The model under review builds one solid part; all positions refer to its coordinate system, in mm. Round coordinates to 2 decimals unless told otherwise and drop trailing zeros. Order: outer loops, then holes, each group sorted by start corner. A loop starts at its lowest first (then second) coordinate and runs counter-clockwise, first axis right, second up. Notation, with made-up numbers: (87, 46.5) - (119, 46.5) arc R13 cw to (119, 65.5) - close; hole circle Ø8 at (-11, -6.75). An arc over 180 degrees is marked (long way). One line per question, with ' | ' between items. Start each with the question number.
Item 1: Add section B-B on z = 19.5. State the section outline as (x, y) points.
Item 2: For L1, parallel to Z at x = 4, y = 187.5 (3 decimals); L2, parallel to X at y = 184.5, z = 3; L3, parallel to X at y = 319, z = 8, list the stretches that pass through material, from the lowest coordinate up. Write a range as [from, to].
Item 3: Insertion check: pin 1 Ø5 at (y, z) = (121.5, 12.5) entering from -X. The pin has a flat end and moves straight along its axis. Give the tip position at first contact, or say it passes through.
Item 4: Add section C-C on y = 136. State the section outline as (x, z) points (3 decimals).
Item 5: Add section A-A on y = 100. State the section outline as (x, z) points (3 decimals).
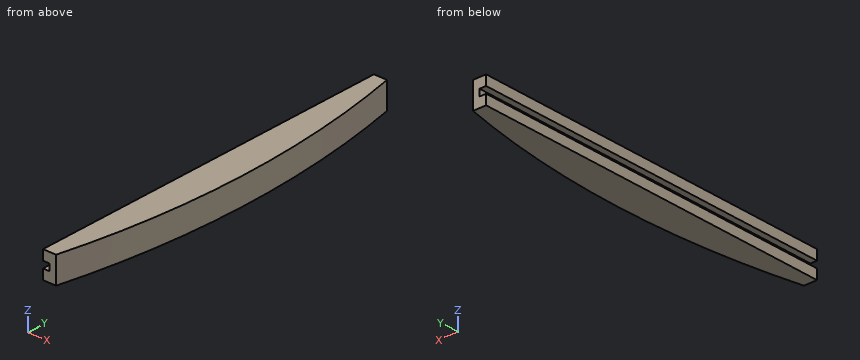
Autodesk Inventor part; units mm, degrees
ref_plane "YZ Plane" through (0, 0, 0) normal (1, 0, 0) x (0, 1, 0)
ref_plane "XZ Plane" through (0, 0, 0) normal (0, 1, 0) x (-1, 0, 0)
ref_plane "XY Plane" through (0, 0, 0) normal (0, 0, 1) x (1, 0, 0)
sketch "Sketch1" plane through (0, 0, 0) normal (0, 0, 1) x (1, 0, 0)
  line L0 (0, 0) -> (12.7, 0)
  line L1 (0, 0) -> (0, 355.8819)
  line L2 (0, 355.8819) -> (12.7, 355.8819)
  arc A0 (12.7, 0) -> (12.7, 355.8819) centre (-782.8431, 177.941) ccw
  dimension "d0" = 12.7
  dimension "d1" = 355.8819
  dimension "d2" = 12.7
extrude "Extrusion1" add sketch "Sketch1" along normal blind 25.4
sketch "Sketch2" plane through (0, 0, 0) normal (-1, 0, 0) x (0, 0, 1)
  line L0 (0, 0) -> (12.7, 0)
  line L1 (0, 0) -> (25.4, 0)
  line L2 (12.7, 355.8819) -> (9.525, 355.8819)
  line L3 (9.525, 355.8819) -> (9.525, 0)
  line L4 (9.525, 0) -> (15.875, 0)
  line L5 (15.875, 0) -> (15.875, 355.8819)
  line L6 (9.525, 355.8819) -> (15.875, 355.8819)
  line L7 (9.525, 0) -> (15.875, 0)
  dimension "d5" = 12.7
  dimension "d6" = 3.175
  dimension "d7" = 6.35
extrude "Extrusion2" cut sketch "Sketch2" against normal blind 6.35
sketch "Sketch3" plane through (0, 355.8819, 0) normal (0, 1, 0) x (1, 0, 0)
  line L0 (12.7, -25.4) -> (0, -25.4)
  line L1 (12.7, 0) -> (0, 0)
  line L2 (0, -9.525) -> (6.35, -9.525)
  line L3 (6.35, -15.875) -> (0, -15.875)
  line L4 (6.35, -9.525) -> (6.35, -15.875)
  line L5 (0, -15.875) -> (0, -25.4)
  line L6 (12.7, 0) -> (12.7, -25.4)
  point P0 (6.35, 0)
  dimension "d10" = 25.4
  dimension "d11" = 9.525
  dimension "d12" = 6.35
  dimension "d13" = 6.35
  dimension "d14" = 12.7
sketch "Sketch4" plane through (0, 0, 25.4) normal (0, 0, 1) x (1, 0, 0)
  line L0 (12.7, 355.8819) -> (0, 355.8819)
  line L1 (0, 0) -> (12.7, 0)
  dimension "d15" = 355.8819
properties part number "sidestrip_Ocampo"
Determined:
1) outline: (0, 0) - (12.7, 0) arc R815.2 ccw to (12.7, 355.88) - (0, 355.88) - close
2) L1: [0, 9.525], [15.875, 25.4] | L2: [0, 32.33] | L3: [0, 20.06]
3) pin 1: x = 6.35
4) outline: (0, 0) - (31.278, 0) - (31.278, 25.4) - (0, 25.4) - (0, 15.875) - (6.35, 15.875) - (6.35, 9.525) - (0, 9.525) - close
5) outline: (0, 0) - (28.623, 0) - (28.623, 25.4) - (0, 25.4) - (0, 15.875) - (6.35, 15.875) - (6.35, 9.525) - (0, 9.525) - close
